from build123d import *

# Parameters (mm, degrees)
BOSS_EXTRUDE1_DEPTH = 48.26
SKETCH3_R           = 12.446
CUT_EXTRUDE1_DEPTH  = 44.196
SKETCH4_R           = 3.175
CUT_EXTRUDE2_DEPTH  = 40.64


with BuildPart() as part:
    # Sketch2 → Boss-Extrude1 (new body)
    with BuildSketch(Plane.XY):
        with BuildLine():
            Line((-14.986, 0), (-14.986, 101.6))
            Line((-14.986, 101.6), (14.986, 101.6))
            Line((14.986, 101.6), (14.986, 0))
            ThreePointArc((14.986, 0), (0, -14.986), (-14.986, 0))
        make_face()
    extrude(amount=BOSS_EXTRUDE1_DEPTH)

    # Sketch3 → Cut-Extrude1 (cut)
    with BuildSketch(Plane.XY.offset(48.26)):
        Circle(SKETCH3_R)
    extrude(amount=-CUT_EXTRUDE1_DEPTH, mode=Mode.SUBTRACT)

    # Sketch4 → Cut-Extrude2 (cut)
    with BuildSketch(Plane(origin=(0, 0, 0), x_dir=(-1, 0, 0), z_dir=(0, 0, -1))):
        Circle(SKETCH4_R)
    extrude(amount=-CUT_EXTRUDE2_DEPTH, mode=Mode.SUBTRACT)


solid = part.part
Read the model definition and answer for the solid it produces. Units are mm, in the model's axes. Give positions to 0.01 mm unless a question says otherwise; leave off trailing zeros. Write each loop counter-clockwise with the first axis right and the second up, starting at its lowest first coordinate (ties: lowest second). Pieces come first, ordered by that corner, then holes. Notation, with made-up numbers: (11.5, -35) - (31.5, -35) arc R34 cw to (31.5, -3) - close; hole circle Ø6 at (38, -32.5). An arc over 180 degrees is marked (long way). Answer in a Markdown table with one row per item. Add a question column.
Item 1: Find the intervals of material crossed by L1, parallel to Y at x = 0, z = 37; L2, parallel to Y at x = 0, z = 1.7 (3 decimals); L3, parallel to Z at x = 8.25, y = -5, in increasing order.
Item 2: Section C-C, the plane x = -6.25 is taken. Write down the section's boundary in (y, z), and give its area (3 significant figures).
Item 3: Section A-A, the plane x = 0 is taken. Write down the section's boundary in (y, z) (3 decimals), and give its area (3 significant figures).
Item 4: Determine the mould class of faces 1 (the face through (-2.7, -12.15, 26.47)), 2 (the face through (0, 101.6, 24)), 3 (the face through (14.986, 52, 24)), 4 (the face through (3, -3, 4.064)) for opening direction Y: pulls with the +Y half, pulls with the -Y half, needs draft (parallel to the pull), parting line crosses it, or undercut.
Item 5: Flat-ended cylindrical pins translate along their axes: P1, Ø1, axis at x = -4.5, z = 18.5, coming from the -Y side; P2, Ø7.5, axis at x = 0, y = 0, coming from the +Z side. Find the tip coordinate at first contact, or state that the pin passes through.
Item 6: Section B-B, the plane z = 22 is taken. Write down the section's boundary in (x, y).
Recorded:
| question | item | result |
|---|---|---|
| 1 | L1 | y = -14.99 to -12.45, 12.45 to 101.6 |
| 1 | L2 | y = -14.986 to -3.175, 3.175 to 101.6 |
| 1 | L3 | z = 0 to 4.06 |
| 2 | outline | (-13.62, 0) - (101.6, 0) - (101.6, 48.26) - (10.76, 48.26) - (10.76, 4.06) - (-10.76, 4.06) - (-10.76, 48.26) - (-13.62, 48.26) - close |
| 2 | area | 4,610 mm2 |
| 3 | outline | (-14.986, 0) - (-3.175, 0) - (-3.175, 4.064) - (-12.446, 4.064) - (-12.446, 48.26) - (-14.986, 48.26) - close; (3.175, 0) - (101.6, 0) - (101.6, 48.26) - (12.446, 48.26) - (12.446, 4.064) - (3.175, 4.064) - close |
| 3 | area | 4,500 mm2 |
| 4 | face 1 | undercut |
| 4 | face 2 | pulls with the +Y half |
| 4 | face 3 | needs draft |
| 4 | face 4 | undercut |
| 5 | P1 | stops at y = -14.44 |
| 5 | P2 | stops at z = 4.06 |
| 6 | outline | (-14.99, 0) arc R14.99 ccw to (14.99, 0) - (14.99, 101.6) - (-14.99, 101.6) - close; hole circle Ø24.89 at (0, 0) |
